Work out the finished part from the listing and answer in its coordinate system (mm). Face numbers are marked on the shaded views. A direction names the side the tool comes from. Give positions to 0.01 mm unless a question says otherwise; leave off trailing zeros. Loops run counter-clockwise (first coordinate to the right, second up) from the corner with the lowest first, then second, coordinate; pieces in that order, holes last. Notation, with made-up numbers: (89, 39.5) - (107, 39.5) arc R19 cw to (107, 70.5) - close; hole circle Ø4 at (-13.75, 43). An arc over 180 degrees is marked (long way). One line per question, with ' | ' between items.
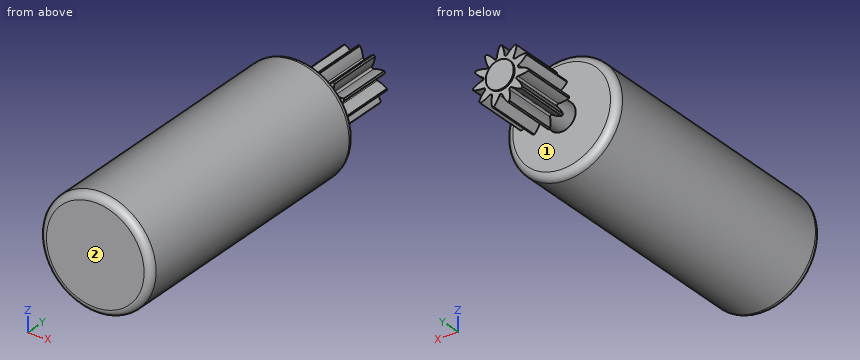
from build123d import *

# Parameters (mm, degrees)
FILLET1_R          = 0.5
CUT_EXTRUDE1_DEPTH = 4
CIRPATTERN1_COUNT  = 11


with BuildPart() as part:
    # Sketch3 → Revolve1 (revolve)
    with BuildSketch(Plane.XY):
        Polygon((0, 0), (0, 26.1), (1, 26.1), (1, 26), (2, 26), (2, 22), (1, 22), (1, 20), (4, 20), (4, 0), align=None)
    revolve(axis=Axis((0, 0, 0), (0, 1, 0)))

    # Fillet1
    fillet1_edges = [part.edges().sort_by_distance(p)[0] for p in [
        (-4, 20, 0),
        (-4, 0, 0),
    ]]
    fillet(fillet1_edges, radius=FILLET1_R)

    # Sketch4 → Cut-Extrude1 (cut)
    with BuildSketch(Plane(origin=(0, 26, 0), x_dir=(1, 0, 0), z_dir=(0, 1, 0))):
        with BuildLine():
            ThreePointArc((-0.5, 1.936491673), (-0.266119458, 1.637619869), (-0.092905413, 1.299949383))
            ThreePointArc((-0.092905413, 1.299949383), (0, 1.236943764), (0.092905413, 1.299949383))
            ThreePointArc((0.092905413, 1.299949383), (0.266119458, 1.637619869), (0.5, 1.936491673))
            ThreePointArc((0.5, 1.936491673), (0, 2), (-0.5, 1.936491673))
        make_face()
    cut_extrude1 = extrude(amount=-CUT_EXTRUDE1_DEPTH, mode=Mode.SUBTRACT)

    # CirPattern1: Cut-Extrude1 ×11 about axis
    cirpattern1_axis = Axis((0, 0, 0), (0, 1, 0))
    for i in range(1, CIRPATTERN1_COUNT):
        add(cut_extrude1.rotate(cirpattern1_axis, i * 360 / CIRPATTERN1_COUNT), mode=Mode.SUBTRACT)


solid = part.part
1. Find section A-A on y = 12.75. Write down the section's boundary in (x, z), then the cut area to 3 significant figures.
Evaluation:
outline: circle Ø8 at (0, 0) | area: 50.3 mm2
2. Flat-ended cylindrical pins translate along their axes: pin 1 (1.5 mm diameter, centred on x = 2, z = 2.5, fed in from +Y); pin 2 (1.5 mm diameter, centred on x = -1, y = 4.5, fed in from -Z); pin 3 (1 mm diameter, centred on y = 4, z = 1, fed in from -X). Find the tip coordinate at first contact, or state that the pin passes through.
Evaluation:
pin 1: y = 20 | pin 2: z = -3.99 | pin 3: x = -3.97
3. Consider L1, parallel to Y at x = 1.25, z = -1.25; L2, parallel to Y at x = -2.25, z = -2; L3, parallel to Z at x = -1.75, y = 22.25. Determine where each line is inside the solid, lowest interval first.
Evaluation:
L1: 0 to 20, 22 to 26 | L2: 0 to 20 | L3: -0.41 to -0.07, 0.66 to 0.89
4. Which of the six approach directions +Z, -Z, +X, -X, +Y, -Y give full straight-line access (tool end or side, diameter ignored) to the marked faces 1 and 2?
Evaluation:
face 1: none | face 2: +Z, -Z, +X, -X, -Y
